The listing builds one solid part. Answer for the finished solid, in the listing's coordinates (mm). A direction names the side the tool comes from. Coordinates: 2 decimals unless noted, no trailing zeros. Order: outer loops, then holes, each group sorted by start corner. A loop starts at its lowest first (then second) coordinate and runs counter-clockwise, first axis right, second up. Notation, with made-up numbers: (1.25, 38.25) - (22.25, 38.25) arc R8 cw to (22.25, 49.25) - close; hole circle Ø7 at (10.5, 88.25). An arc over 180 degrees is marked (long way). Use one line per item in the form item = value. Start each with the question number.
Item 1: Consider line 1 along Z through (x, y) = (27, -61) (3 decimals); line 2 along Z through (x, y) = (-1.5, -82.5) (3 decimals). Determine where each line is inside the solid, lowest interval first. Write a range as [from, to].
Item 2: Each of these flat-tipped pins is pushed along its axis until it touches: pin 1 Ø2.5 at (x, z) = (10, 35.5) entering from +Y; pin 2 Ø1 at (x, z) = (-36.5, -15.5) entering from +Y; pin 3 Ø3.5 at (x, z) = (36, 22.5) entering from +Y; pin 4 Ø12 at (x, y) = (-16.5, 10.5) entering from +Z. Where does it stop, or does it pass through?
Item 3: Section B-B, the plane x = 16 is taken. Write down the section's boundary in (y, z) (3 decimals).
Item 4: The mould has two halves that part along Z. Classify faces 1 (the flat face through (18.646, -38.986, 36.535)), 2 (the flat face through (-36.49, 87.736, -12.89)), 3 (the flat face through (6, 12, 38.1)): released by +Z, released by -Z, zero draft, split by the parting line, or undercut.
Item 5: Section A-A, the plane y = 8 is taken. Count the separate pieces of the cut face and the enclosed holes in it, and give its area (3 significant figures).
Item 6: A tool of negligible diameter and unlimited length cuts with its end or side. For faces 4 (the flat face through (38.1, -1, -8)), 5 (the flat face through (-14.44, -41.97, 36.53)), 6 (the flat face through (-36.49, -39.89, 18.96)), from which of +Z, -Z, +X, -X, +Y, -Y can it reach the whole face along a straight path? Write none if from no direction.
from build123d import *

# Parameters (mm, degrees)
F1_DEPTH  = 38.1
F3_W      = 69.85
F3_H      = 69.85
F4_DEPTH  = 127
F5_DEPTH  = 76.2
F7_DEPTH  = 3.175
F8_W      = 6.5186821197
F8_H      = 3.175
F9_DEPTH  = 76.2
F10_W     = 3.175
F10_H     = 190.1626357606
F11_DEPTH = 3.175
F12_DEPTH = 3.2004


with BuildPart() as f1:
    # F0 (on Right) → F1 (new body, symmetric)
    with BuildSketch(Plane.YZ):
        Polygon((-76.2, 38.1), (-101.6, -38.1), (101.6, -38.1), (76.2, 38.1), align=None)
    extrude(amount=F1_DEPTH, both=True)

    # F3 (on Front) → F4 (cut, symmetric)
    with BuildSketch(Plane.XZ):
        Rectangle(F3_W, F3_H)
    extrude(amount=F4_DEPTH, both=True, mode=Mode.SUBTRACT)

    # F2 (on face) → F5 (cut)
    with BuildSketch(Plane.YZ.offset(38.1)):
        Polygon((-95.0813178803, -34.925), (-81.28, -34.925), (-81.28, 6.4789536409), align=None)
        Polygon((-76.2, -29.37570354), (-15.1619292031, -2.54), (-76.2, -2.54), align=None)
        Polygon((-76.2, 2.54), (-15.1619292031, 2.54), (-76.2, 29.37570354), align=None)
        Polygon((-76.2, 34.925), (-2.54, 2.54), (-2.54, 34.925), align=None)
        Polygon((2.54, 34.925), (2.54, 2.54), (76.2, 34.925), align=None)
        Polygon((15.1619292031, 2.54), (76.2, 2.54), (76.2, 29.37570354), align=None)
        Polygon((15.1619292031, -2.54), (76.2, -29.37570354), (76.2, -2.54), align=None)
        Polygon((2.54, -34.925), (76.2, -34.925), (2.54, -2.54), align=None)
        Polygon((81.28, 6.4789536409), (81.28, -34.925), (95.0813178803, -34.925), align=None)
        Polygon((-76.2, -34.925), (-2.54, -34.925), (-2.54, -2.54), align=None)
    extrude(amount=-F5_DEPTH, mode=Mode.SUBTRACT)

    # F6 (on face) → F7 (cut)
    with BuildSketch(Plane.XY.offset(38.1)):
        Polygon((0, 0), (34.925, 73.025), (-34.925, 73.025), align=None)
        Polygon((-34.925, 61.2509003959), (-34.925, -73.025), (-2.8155455575, -5.8870498021), align=None)
        Polygon((2.8155455575, -5.8870498021), (34.925, -73.025), (34.925, 61.2509003959), align=None)
        Polygon((-29.293908885, -73.025), (29.293908885, -73.025), (0, -11.7740996041), align=None)
    extrude(amount=-F7_DEPTH, mode=Mode.SUBTRACT)

    # F8 (on face) → F9 (join)
    with BuildSketch(Plane.YZ.offset(38.1)):
        with Locations((-98.3406589402, -36.5125)):
            Rectangle(F8_W, F8_H)
        with Locations((98.3406589402, -36.5125)):
            Rectangle(F8_W, F8_H)
    extrude(amount=-F9_DEPTH)

    # F10 (on face) → F11 (join)
    with BuildSketch(Plane.XY.offset(-34.925)):
        with Locations((36.5125, 0)):
            Rectangle(F10_W, F10_H)
        with Locations((-36.5125, 0)):
            Rectangle(F10_W, F10_H)
    extrude(amount=F11_DEPTH)

    # F10 (on face) → F12 (join)
    with BuildSketch(Plane.XY.offset(-34.925)):
        with Locations((36.5125, 0)):
            Rectangle(F10_W, F10_H)
        with Locations((-36.5125, 0)):
            Rectangle(F10_W, F10_H)
    extrude(amount=F12_DEPTH)


solid = f1.part
Response:
q1.line_1 = [-38.1, -34.925], [34.925, 38.1]
q1.line_2 = [-38.1, -34.925]
q2.pin_1 = 77.26
q2.pin_2 = 94.23
q2.pin_3 = 81.98
q2.pin_4 = 38.1
q3.outline = (-101.6, -38.1) - (101.6, -38.1) - (101.6, -34.925) - (-101.6, -34.925) - close; (-77.258, 34.925) - (-73.025, 34.925) - (-73.025, 38.1) - (-76.2, 38.1) - close; (-45.229, 34.925) - (-33.455, 34.925) - (-33.455, 38.1) - (-45.229, 38.1) - close; (21.68, 34.925) - (33.455, 34.925) - (33.455, 38.1) - (21.68, 38.1) - close; (73.025, 34.925) - (77.258, 34.925) - (76.2, 38.1) - (73.025, 38.1) - close
q4.face_1 = zero draft
q4.face_2 = undercut
q4.face_3 = released by +Z
q5.separate_pieces = 7
q5.enclosed_holes = 0
q5.area = 381 mm2
q6.face_4 = +Z, -Z, +X, +Y, -Y
q6.face_5 = +Z
q6.face_6 = +X, -X
